from build123d import *

# Parameters (mm, degrees)
F1_DEPTH  = 1.524
F3_DEPTH  = 5.588
F4_R      = 1.4605
F5_DEPTH  = 1.143
F7_SIZE   = 0.508
F9_DEPTH  = 0.3175
F11_ANGLE = 90
F13_ANGLE = 180
F15_W     = 1.2032650411
F15_H     = 6.585133262
F15_W_2   = 0.635
F15_H_2   = 0.508
F16_DEPTH = 1.524
F17_R     = 1.524
F18_DEPTH = 25.4


# Not quite as in the source:
# - a fillet or chamfer that OpenCascade refuses, or shapes differently, is made with other operations: its cross-section is extruded or revolved along the edge and cut away or added


with BuildPart() as f1:
    # F0 (on Top) → F1 (new body)
    with BuildSketch(Plane.XY):
        Polygon((-17.78, -5.08), (13.97, -5.08), (16.4832153797, -2.5667846203), (7.62, -2.5667846203), (7.62, 2.5667846203), (16.4832153797, 2.5667846203), (13.97, 5.08), (-17.78, 5.08), align=None)
        Polygon((7.62, -2.5667846203), (16.4832153797, -2.5667846203), (17.78, -1.27), (17.78, 1.27), (16.4832153797, 2.5667846203), (7.62, 2.5667846203), align=None)
    extrude(amount=-F1_DEPTH)

    # F2 (on face) → F3 (join)
    with BuildSketch(Plane.XY):
        Polygon((16.4832153797, -2.5667846203), (17.78, -1.27), (17.78, 1.27), (16.4832153797, 2.5667846203), (7.62, 2.5667846203), (7.62, -2.5667846203), align=None)
    extrude(amount=F3_DEPTH)

    # F4 (on face) → F5 (join)
    with BuildSketch(Plane.XY.offset(5.588)):
        with Locations((10.829353705, 0)):
            Circle(F4_R)
        with Locations((14.7973923013, 0)):
            Circle(F4_R)
    extrude(amount=F5_DEPTH)

    # F6: fillet of radius 1.27 on 2 edges, made by hand

    # F6_s1 → F6_t2 (revolve, cut)
    with BuildSketch(Plane.XZ):
        with BuildLine():
            ThreePointArc((12.289853705, 5.588), (11.8781615594, 6.4028572079), (11.0262196599, 6.731))
            Line((11.0262196599, 6.731), (12.289853705, 6.731))
            Line((12.289853705, 6.731), (12.289853705, 5.588))
        make_face()
    revolve(axis=Axis((10.829353705, 0, 6.731), (0, 0, 1)), mode=Mode.SUBTRACT)

    # F6_s3 → F6_t4 (revolve, cut)
    with BuildSketch(Plane.XZ):
        with BuildLine():
            ThreePointArc((16.2578923013, 5.588), (15.8462001556, 6.4028572079), (14.9942582561, 6.731))
            Line((14.9942582561, 6.731), (16.2578923013, 6.731))
            Line((16.2578923013, 6.731), (16.2578923013, 5.588))
        make_face()
    revolve(axis=Axis((14.7973923013, 0, 6.731), (0, 0, 1)), mode=Mode.SUBTRACT)

    # F7
    f7_edges = [f1.edges().sort_by_distance(p)[0] for p in [
        (12.051608, -2.566785, 5.588),
        (12.051608, 2.566785, 5.588),
        (7.62, 0, 5.588),
        (17.78, 0, 5.588),
        (17.131608, -1.918392, 5.588),
        (17.131608, 1.918392, 5.588),
    ]]
    chamfer(f7_edges, length=F7_SIZE)

    # F12: F10_1 across plane


with BuildPart() as f9:
    # F8 (on Front) → F9 (new body, symmetric)
    with BuildSketch(Plane.XZ):
        with BuildLine():
            Line((-22.86, -5.334), (-22.86, -5.842))
            Line((-22.86, -5.842), (-15.9157037269, -5.842))
            ThreePointArc((-15.9157037269, -5.842), (-15.5230394847, -5.6793531454), (-15.3603926301, -5.2866889032))
            Line((-15.3603926301, -5.2866889032), (-15.3603926301, -1.1672781548))
            Line((-15.3603926301, -1.1672781548), (-15.8683926301, -1.1672781548))
            Line((-15.8683926301, -1.1672781548), (-15.8683926301, -5.334))
            Line((-15.8683926301, -5.334), (-22.86, -5.334))
        make_face()
    extrude(amount=F9_DEPTH, both=True)


with BuildPart() as f10_1:
    # F10: copy of F9
    add(f9.part.moved(Location((0, -2.92, 0))))


with BuildPart() as f10_1_1:
    # F11: moved
    add(f10_1.part.rotate(Axis((-15.8683926301, -2.6025, -3.2506390774), (0, 0, 1)), F11_ANGLE))


with BuildPart() as f1_1:
    add(f1.part)
    add(f10_1_1.part.mirror(Plane.XZ))



with BuildPart() as f9_1:
    # F13: moved
    add(f9.part.rotate(Axis((-15.8683926301, 0.3175, -3.2506390774), (0, 0, 1)), F13_ANGLE))


with BuildPart() as f9_2:
    # F14: moved
    add(f9_1.part.moved(Location((0.635, -0.635, 0))))


with BuildPart() as f1_2:
    add(f1_1.part)

    add(f9_2.part)  # F16 merges F9

    add(f10_1_1.part)  # F16 merges F10_1
    # F15 (on face) → F16 (join)
    with BuildSketch(Plane(origin=(0, 0, -1.524), x_dir=(1, 0, 0), z_dir=(0, 0, -1))):
        with Locations((-15.6205464154, 0)):
            Rectangle(F15_W, F15_H)
        with Locations((-15.5508926301, -2.3485)):
            Rectangle(F15_W_2, F15_H_2, mode=Mode.SUBTRACT)
    extrude(amount=F16_DEPTH)

    # F17 (on face) → F18 (cut)
    with BuildSketch(Plane(origin=(0, 0, -1.524), x_dir=(1, 0, 0), z_dir=(0, 0, -1))):
        with Locations((-0.254, 0)):
            Circle(F17_R)
    extrude(amount=-F18_DEPTH, mode=Mode.SUBTRACT)


solid = f1_2.part
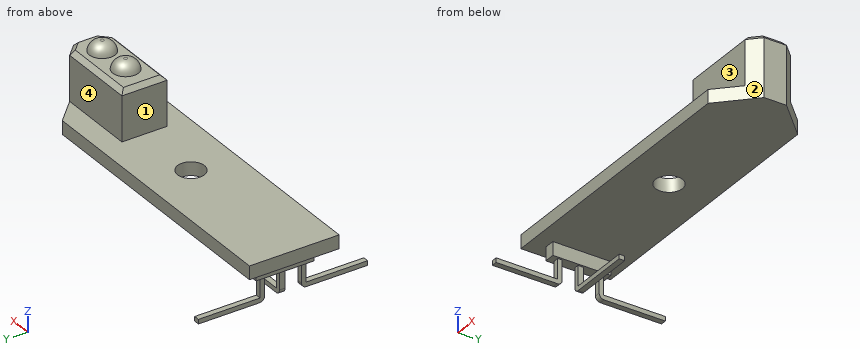
The model under review builds one solid part; all positions refer to its coordinate system, in mm. Face numbers are marked on the shaded views. A direction names the side the tool comes from. Round coordinates to 2 decimals unless told otherwise and drop trailing zeros. Order: outer loops, then holes, each group sorted by start corner. A loop starts at its lowest first (then second) coordinate and runs counter-clockwise, first axis right, second up. Notation, with made-up numbers: (86, -29.5) -> (108, -29.5) arc R9 cw to (108, -18.5) -> close; hole circle Ø9 at (-19, 85). An arc over 180 degrees is marked (long way). Return JSON: item names as keys, results as strings.
1. For the marked faces 1, 2, 3 and 4, list the 3-axis set-ups (+Z, -Z, +X, -X, +Y, -Y) from which the entire face can be reached by the end or side of a thin tool; tool diameter is ignored.
Answer block:
{"face 1": "+Z, -X, +Y, -Y", "face 2": "+Z, -Z, +X, -Y", "face 3": "+Z, +X, -X, -Y", "face 4": "+Z, +X, -X, +Y"}
2. Take a section at A-A (x = -14). Write out the cut boundary in (y, z).
Answer block:
{"outline": "(-5.08, -1.52) -> (5.08, -1.52) -> (5.08, 0) -> (-5.08, 0) -> close; (-0.32, -5.84) -> (0.32, -5.84) -> (0.32, -5.33) -> (-0.32, -5.33) -> close"}
3. Take a section at B-B (y = -4). Write out the cut boundary in (x, z).
Answer block:
{"outline": "(-17.78, -1.52) -> (15.05, -1.52) -> (15.05, 0) -> (-17.78, 0) -> close; (-15.87, -5.84) -> (-15.23, -5.84) -> (-15.23, -5.33) -> (-15.87, -5.33) -> close"}
4. Take a section at D-D (x = -3.5). Write out the cut boundary in (y, z).
Answer block:
{"outline": "(-5.08, -1.52) -> (5.08, -1.52) -> (5.08, 0) -> (-5.08, 0) -> close"}
5. For L1, parallel to X at y = 0, z = -1; L2, parallel to Z at x = -7.5, y = 3.5; L3, parallel to X at y = 1, z = 3.25, list the stretches that pass through material, from the lowest coordinate up. Write a range as [from, to].
Answer block:
{"L1": "x = [-17.78, -1.78], [1.27, 17.78]", "L2": "z = [-1.52, 0]", "L3": "x = [7.62, 17.78]"}
6. Take a section at C-C (z = 4.5). Write out the cut boundary in (x, y).
Answer block:
{"outline": "(7.62, -2.57) -> (16.48, -2.57) -> (17.78, -1.27) -> (17.78, 1.27) -> (16.48, 2.57) -> (7.62, 2.57) -> close"}
7. Insertion check: P1, Ø1, axis at x = 12, z = 2.5, coming from the +Y side; P2, Ø0.5, axis at y = 0, z = -2.5, coming from the -X side; P3, Ø0.6, axis at x = -15.5, z = -2.5, coming from the -Y side; P4, Ø2.5, axis at x = -0.254, y = 0, coming from the -Z side. Each pin has a flat end and moves straight along its axis. Give the tip position at first contact, or say it passes through.
Answer block:
{"P1": "stops at y = 2.57", "P2": "stops at x = -16.22", "P3": "stops at y = -3.29", "P4": "passes through"}
